The model under review builds one solid part; all positions refer to its coordinate system, in mm. Face numbers are marked on the shaded views. A direction names the side the tool comes from. Coordinates: 2 decimals unless noted, no trailing zeros. Write each loop counter-clockwise with the first axis right and the second up, starting at its lowest first coordinate (ties: lowest second). Pieces come first, ordered by that corner, then holes. Notation, with made-up numbers: (-35, -5) - (2, -5) arc R24 cw to (2, 5) - close; hole circle Ø4 at (46.25, 20.25). An arc over 180 degrees is marked (long way). Return JSON: item names as keys, results as strings. Group by question number.
(1) Tool access review of the marked faces 4, 5 and 6: name each direction out of +Z, -Z, +X, -X, +Y, -Y from which nothing blocks a thin tool from reaching the whole face with its end or side.
(2) We need section A-A on z = 6.05. Give the number of separate pieces and of enclosed holes in the cut face, then the cut area to 3 significant figures.
(3) For pin 1 Ø1 at (x, y) = (41, 40) entering from +Z; pin 2 Ø1.5 at (x, y) = (48, 40) entering from -Z; pin 3 Ø1 at (x, y) = (58, 40) entering from -Z; pin 4 Ø1 at (y, z) = (40.5, 6.5) entering from +X, all flat-tipped, find the tip position at first contact; note any pin that passes through.
(4) Draft analysis for pull direction X (two halves, no side actions). For the marked faces 1, 2 and 3, state which applies: released by +X, released by -X, zero draft, split by the parting line, or undercut.
(5) To check wall thickness, follow L1, parallel to X at y = 41.2, z = 6.55; L2, parallel to X at y = 41.6, z = 6.6; L3, parallel to X at y = 39.3, z = 5.4. State the ranges of each line that lie inside material, in increasing order. Write a range as from..to.
(6) We need section B-B on x = 47. State the section outline as (y, z) points, then the cut area to 3 significant figures.
```python
from build123d import *

# Parameters (mm, degrees)
PAD011_DEPTH               = 4
PAD011_MIRRORED008_2_DEPTH = 4
LINEARPATTERN004_COUNT     = 2
LINEARPATTERN004_PITCH     = 6.5
SKETCH041_W                = 2
SKETCH041_H                = 0.4
PAD022_DEPTH               = 4


with BuildPart() as part:
    # Sketch024 (on DatumPlane) → Pad011 (new body)
    with BuildSketch(Plane(origin=(55, 42.304, 0), x_dir=(1, 0, 0), z_dir=(0, -1, 0))):
        with BuildLine():
            Line((0, 5.2), (0, 5.6))
            ThreePointArc((0, 5.6), (0.125164, 5.6132), (0.24482, 5.65222))
            Line((0.24482, 5.65222), (2.841966, 6.812967))
            ThreePointArc((3.25, 6.9), (3.041394, 6.878), (2.841966, 6.812967))
            Line((3.25, 6.5), (3.25, 6.9))
            ThreePointArc((3.25, 6.5), (3.124841, 6.486801), (3.005188, 6.447784))
            Line((0.408034, 5.287033), (3.005188, 6.447784))
            ThreePointArc((0, 5.2), (0.208606, 5.222), (0.408034, 5.287033))
        make_face()
    pad011 = extrude(amount=PAD011_DEPTH)

    # Sketch024 Mirrored008 2 → Pad011 Mirrored008 2 (add)
    with BuildSketch(Plane(origin=(61.5, 42.304, 0), x_dir=(-1, 0, 0), z_dir=(0, 1, 0))):
        with BuildLine():
            Line((0, 5.2), (0, 5.6))
            ThreePointArc((0, 5.6), (0.125164, 5.6132), (0.24482, 5.65222))
            Line((0.24482, 5.65222), (2.841966, 6.812967))
            ThreePointArc((3.25, 6.9), (3.041394, 6.878), (2.841966, 6.812967))
            Line((3.25, 6.5), (3.25, 6.9))
            ThreePointArc((3.25, 6.5), (3.124841, 6.486801), (3.005188, 6.447784))
            Line((0.408034, 5.287033), (3.005188, 6.447784))
            ThreePointArc((0, 5.2), (0.208606, 5.222), (0.408034, 5.287033))
        make_face()
    pad011_mirrored008_2 = extrude(amount=-PAD011_MIRRORED008_2_DEPTH)

    # LinearPattern004: Pad011, Pad011 Mirrored008 2 ×2
    with Locations(*[(i * LINEARPATTERN004_PITCH, 0, 0) for i in range(1, LINEARPATTERN004_COUNT)]):
        add(pad011)
        add(pad011_mirrored008_2)

    # Sketch041 (on DatumPlane) → Pad022 (join)
    with BuildSketch(Plane(origin=(55, 42.304, 0), x_dir=(1, 0, 0), z_dir=(0, -1, 0))):
        with Locations((14, 5.4)):
            Rectangle(SKETCH041_W, SKETCH041_H)
    extrude(amount=PAD022_DEPTH)

    # Mirrored009: part across Sketch041 V_Axis


with BuildPart() as part_1:
    add(part.part)
    add(part.part.mirror(Plane(origin=(55, 42.304, 0), x_dir=(0, -1, 0), z_dir=(1, 0, 0))))


solid = part_1.part
```
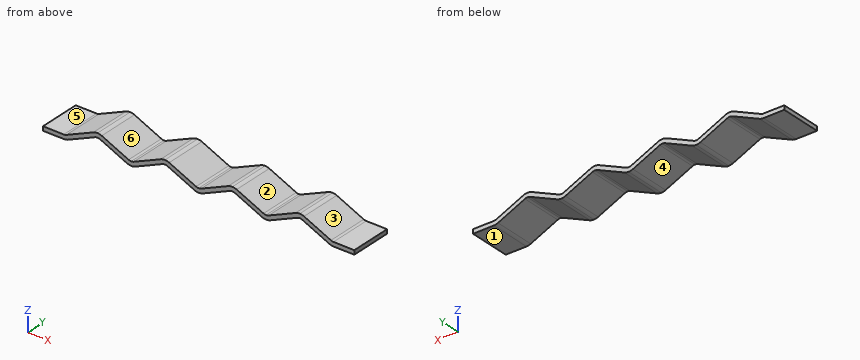
Ans:
{
 "1": {"face 4": "-Z, +Y, -Y", "face 5": "+Z, -X, +Y, -Y", "face 6": "+Z, +Y, -Y"},
 "2": {"separate pieces": "8", "enclosed holes": "0", "area": "31.4 mm²"},
 "3": {"pin 1": "z = 5.6", "pin 2": "z = 5.2", "pin 3": "z = 6.22", "pin 4": "x = 66.98"},
 "4": {"face 1": "zero draft", "face 2": "undercut", "face 3": "released by +X"},
 "5": {"L1": "44.25..46.25, 50.75..52.75, 57.25..59.25, 63.75..65.75", "L2": "44.37..46.13, 50.87..52.63, 57.37..59.13, 63.87..65.63", "L3": "40..42.66, 47.84..49.16, 54.34..55.66, 60.84..62.16, 67.34..70"},
 "6": {"outline": "(38.3, 5.78) - (42.3, 5.78) - (42.3, 6.21) - (38.3, 6.21) - close", "area": "1.75 mm²"}
}
